For this review, take the finished solid that the model builds, in its own axes (mm). A direction names the side the tool comes from. Give positions to 0.01 mm unless a question says otherwise; leave off trailing zeros. Write each loop counter-clockwise with the first axis right and the second up, starting at its lowest first coordinate (ties: lowest second). Pieces come first, ordered by that corner, then holes. Notation, with made-up numbers: M 55,45 L 75,45 A23 cw 75,81 Z; hole C 17.5,-4.5 d5. An arc over 180 degrees is marked long. Use one line per item in the form item = value. Start each with the question number.
Q1. Consider section C-C on y = -4.5. Write out the cut boundary in (x, z), and give its area (3 significant figures).
Q2. Consider section D-D on z = 116.5. Write out the cut boundary in (x, y), and give its area (3 significant figures).
Q3. Consider section B-B on x = -6.5. Write out the cut boundary in (y, z).
Q4. Clearance check with flat-ended pins moving along their axes: pin 1 Ø3 at (x, z) = (-8.5, 122) entering from -Y; pin 2 Ø1.2 at (y, z) = (-44, 59) entering from -X; pin 3 Ø5 at (x, y) = (-17.5, -17) entering from -Z. State where each tip first meets the part, or that it passes through.
Q5. Consider section A-A on z = 93. Write out the cut boundary in (x, y), and give its area (3 significant figures).
Q6. Tool access review of faces 1 (the flat face through (1, -6.706, 67)), 2 (the flat face through (-35, -45.52, 67)), 3 (the flat face through (-1.764, -4, 67)): name each direction out of +Z, -Z, +X, -X, +Y, -Y from which nothing blocks a thin tool from reaching the whole face with its end or side.
Q7. Mouldability with a two-part tool opening along Y and no side actions: class faces 4 (the flat face through (-35, -2.734, 67)), 5 (the flat face through (-1, -41.633, 67)), 6 (the flat face through (-31.335, -5, 67)) as released by +Y, released by -Y, zero draft, split by the parting line, or undercut.
Q8. For probe 1 along Y at (x, z) = (-1, 46); probe 2 along Z at (x, y) = (-8, -25); probe 3 along Y at (x, z) = (-33, 75), list the stretches that pass through material, from the lowest coordinate up. Write a range as [from, to].
```python
from build123d import *

# Parameters (mm, degrees)
F1_DEPTH  = 4.1148
F4_W      = 1.7967561726
F4_H      = 11.5752667189
F5_DEPTH  = 25.4
F3_W      = 21.1648978293
F3_H      = 11.7423608899
F6_DEPTH  = 25.4
F7_W      = 21.1648978293
F7_H      = 7.5958641246
F8_DEPTH  = 25.4
F9_DEPTH  = 25.4
F10_DEPTH = 25.4
F11_W     = 5.1620183513
F11_H     = 4.3984993827
F11_W_2   = 6.7732334137
F11_H_2   = 3.9715627208
F11_W_3   = 4.8598810099
F11_H_3   = 5.2507780492
F11_W_4   = 4.6935081482
F11_H_4   = 3.8872100413
F12_DEPTH = 59.69
F13_DEPTH = 4.826


with BuildPart() as f1:
    # F0 (on Front) → F1 (new body)
    with BuildSketch(Plane.XZ):
        Polygon((1.2734923512, 7.3978709988), (1.0500258068, 4.5483880676), (11.4485891536, 4.5483880676), (12.1993478388, 7.3978709988), align=None)
        Polygon((-2.1805709694, 3.6492620129), (1.0500258068, 4.5483880676), (1.2734923512, 7.3978709988), (-2.1805709694, 6.1951475218), align=None)
        Polygon((11.4485891536, 4.5483880676), (1.0500258068, 4.5483880676), (-2.1805709694, 3.6492620129), (-0.5589149077, 2.3352366406), (16.0257890821, 2.3352366406), align=None)
        Polygon((12.1993478388, 7.3978709988), (11.4485891536, 4.5483880676), (16.0257890821, 2.3352366406), (17.6053401083, 4.832720384), align=None)
    extrude(amount=F1_DEPTH)


with BuildPart() as f5:
    # F4 (on face) → F5 (new body)
    with BuildSketch(Plane.XZ):
        with Locations((4.1603924474, 102.1747291088)):
            Rectangle(F4_W, F4_H)
    extrude(amount=F5_DEPTH)

    # F3 (on Front) → F6 (join)
    with BuildSketch(Plane.XZ):
        with Locations((-5.4645147175, 102.1133996546)):
            Rectangle(F3_W, F3_H)
    extrude(amount=F6_DEPTH)

    # F7 (on face) → F8 (join)
    with BuildSketch(Plane.XY.offset(107.9845800996)):
        with Locations((-5.4645147175, -3.7979320623)):
            Rectangle(F7_W, F7_H)
    extrude(amount=F8_DEPTH)

    # F9 (add): a face of the model
    f9_faces = [f5.faces().sort_by_distance(p)[0] for p in [
        (-5.4645147175, -25.4, 102.1133996546),
    ]]
    extrude(f9_faces, amount=F9_DEPTH)

    # F10 (add): a face of the model
    f10_faces = [f5.faces().sort_by_distance(p)[0] for p in [
        (-16.0469636321, -20.1206151979, 106.6520580868),
    ]]
    extrude(f10_faces, amount=F10_DEPTH)

    # F11 (on face) → F12 (join)
    with BuildSketch(Plane(origin=(0, 0, 96.2422192097), x_dir=(1, 0, 0), z_dir=(0, 0, -1))):
        with Locations((0.8170665242, 4.5063399011)):
            Rectangle(F11_W, F11_H)
        with Locations((-34.7215011716, 4.719808232)):
            Rectangle(F11_W_2, F11_H_2)
        with Locations((-0.8347902913, 44.2584287375)):
            Rectangle(F11_W_3, F11_H_3)
        with Locations((-34.7008481622, 43.5766447335)):
            Rectangle(F11_W_4, F11_H_4)
    extrude(amount=F12_DEPTH)

    # F13 (add): a face of the model
    f13_faces = [f5.faces().sort_by_distance(p)[0] for p in [
        (-18.1645147175, 0, 114.8133996546),
    ]]
    extrude(f13_faces, amount=F13_DEPTH)


solid = f5.part
```
Working result:
q1.outline = M -41.45,96.24 L -38.11,96.24 L -38.11,36.55 L -31.33,36.55 L -31.33,96.24 L -1.76,96.24 L -1.76,36.55 L 3.4,36.55 L 3.4,96.24 L 5.12,96.24 L 5.12,133.38 L -41.45,133.38 Z
q1.area = 2,440 mm²
q2.outline = M -41.45,-7.6 L 5.12,-7.6 L 5.12,4.83 L -41.45,4.83 Z
q2.area = 578 mm²
q3.outline = M -50.8,96.24 L 4.83,96.24 L 4.83,133.38 L -7.6,133.38 L -7.6,107.98 L -50.8,107.98 Z
q4.pin_1 = -7.6
q4.pin_2 = -37.05
q4.pin_3 = 96.24
q5.outline = M -38.11,-6.71 L -31.33,-6.71 L -31.33,-2.73 L -38.11,-2.73 Z; M -37.05,-45.52 L -32.35,-45.52 L -32.35,-41.63 L -37.05,-41.63 Z; M -3.26,-46.88 L 1.6,-46.88 L 1.6,-41.63 L -3.26,-41.63 Z; M -1.76,-6.71 L 3.4,-6.71 L 3.4,-2.31 L -1.76,-2.31 Z
q5.area = 93.4 mm²
q6.face_1 = -Z, +X, -X
q6.face_2 = -Z, -X, -Y
q6.face_3 = -Z, +Y
q7.face_4 = released by +Y
q7.face_5 = undercut
q7.face_6 = zero draft
q8.probe_1 = [-46.88, -41.63], [-6.71, -2.31]
q8.probe_2 = [96.24, 107.98]
q8.probe_3 = [-45.52, -41.63], [-6.71, -2.73]
